Design review of the part shown in the three views and the two pictorial views. Dimensions are in mm from the part's minimum x, y and z. Round coordinates to 2 decimals unless told otherwise and drop trailing zeros. Write each loop counter-clockwise with the first axis right and the second up, starting at its lowest first coordinate (ties: lowest second). Pieces come first, ordered by that corner, then holes. Notation, with made-up numbers: (79.25, 18) - (115.25, 18) arc R25 ccw to (115.25, 57) - close; hole circle Ø8 at (21.25, -9.75). An arc over 180 degrees is marked (long way). Use one line per item in the form item = value.
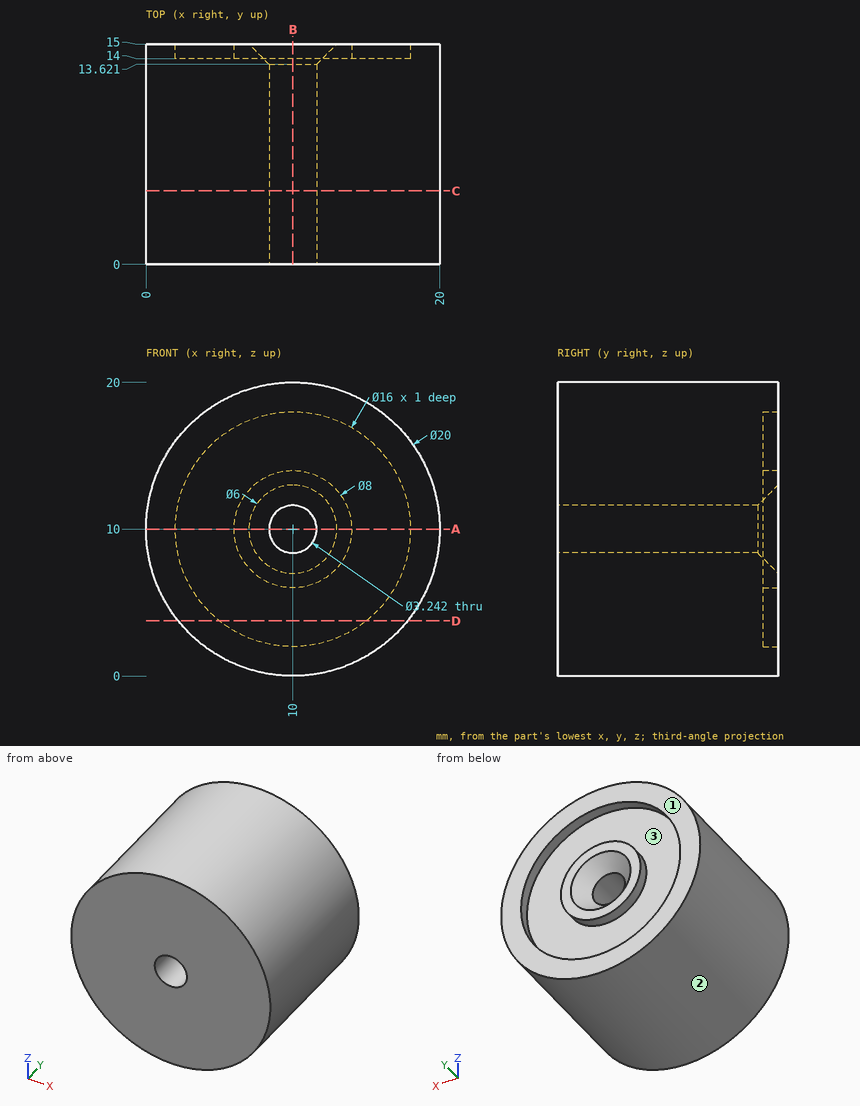
Q1. We need section B-B on x = 10. Write out the cut boundary in (y, z).
Calculated:
outline = (0, 0) - (15, 0) - (15, 2) - (14, 2) - (14, 6) - (15, 6) - (15, 7) - (13.62, 8.38) - (0, 8.38) - close; (0, 11.62) - (13.62, 11.62) - (15, 13) - (15, 14) - (14, 14) - (14, 18) - (15, 18) - (15, 20) - (0, 20) - close
Q2. For P1, Ø12, axis at x = 12, z = 9.5, coming from the -Y side; P2, Ø2, axis at y = 10.5, z = 7, coming from the +X side, all flat-tipped, find the tip position at first contact; note any pin that passes through.
Calculated:
P1 = 0
P2 = 19.8
Q3. To check wall thickness, follow line 1 along Z through (x, y) = (10, 14.55); line 2 along X through (y, z) = (14.75, 6.5); line 3 along Z through (x, y) = (10, 6.5). State the ranges of each line that lie inside material, in increasing order. Write a range as from..to.
Calculated:
line_1 = 0..2, 6..7.45, 12.55..14, 18..20
line_2 = 0.63..2.81, 8.06..11.94, 17.19..19.37
line_3 = 0..8.38, 11.62..20
Q4. Draft analysis for pull direction X (two halves, no side actions). For the marked faces 1, 2 and 3, state which applies: released by +X, released by -X, zero draft, split by the parting line, or undercut.
Calculated:
face_1 = zero draft
face_2 = split by the parting line
face_3 = undercut
Q5. We need section A-A on z = 10. Write out the cut boundary in (x, y).
Calculated:
outline = (0, 0) - (8.38, 0) - (8.38, 13.62) - (7, 15) - (6, 15) - (6, 14) - (2, 14) - (2, 15) - (0, 15) - close; (11.62, 0) - (20, 0) - (20, 15) - (18, 15) - (18, 14) - (14, 14) - (14, 15) - (13, 15) - (11.62, 13.62) - close
Q6. We need section D-D on z = 3.75. Write out the cut boundary in (x, y), then the cut area to 3 significant figures.
Calculated:
outline = (2.19, 0) - (17.81, 0) - (17.81, 15) - (14.99, 15) - (14.99, 14) - (5.01, 14) - (5.01, 15) - (2.19, 15) - close
area = 224 mm2
Q7. We need section C-C on y = 5. Write out the cut boundary in (x, z), then the cut area to 3 significant figures.
Calculated:
outline = circle Ø20 at (10, 10); hole circle Ø3.24 at (10, 10)
area = 306 mm2
